from build123d import *

# Parameters (mm, degrees)
BOSS_EXTRUDE1_DEPTH = 914.4
SKETCH2_W           = 1116.884471925
SKETCH2_H           = 814.4
CUT_EXTRUDE1_DEPTH  = 19950.853735504
BOSS_EXTRUDE3_DEPTH = 850


with BuildPart() as part:
    # Sketch1 → Boss-Extrude1 (new body)
    with BuildSketch(Plane(origin=(0, 0, 0), x_dir=(1, 0, 0), z_dir=(0, 1, 0))):
        with BuildLine():
            Line((-9820.644594144, 1216.884471925), (-9871.125792152, 1216.884471925))
            ThreePointArc((-9871.125792152, 1216.884471925), (-9927.151370921, 609.588288366), (-9945.85, 0))
            Line((-9945.85, 0), (-9895.75, 0))
            ThreePointArc((-9895.75, 0), (-9876.955801384, 609.6), (-9820.644594144, 1216.884471925))
        make_face()
    extrude(amount=BOSS_EXTRUDE1_DEPTH)

    # Sketch2 → Cut-Extrude1 (cut, through all)
    with BuildSketch(Plane(origin=(9945.85, 0, 0), x_dir=(0, 0, -1), z_dir=(1, 0, 0))):
        with Locations((608.442235963, 457.2)):
            Rectangle(SKETCH2_W, SKETCH2_H)
    extrude(amount=-CUT_EXTRUDE1_DEPTH, mode=Mode.SUBTRACT)

    # Sketch5 → Boss-Extrude3 (add)
    with BuildSketch(Plane.XZ.offset(-864.4)):
        Polygon((-9925.583865068, -634.6), (-9875.381051003, -634.6), (-9878.46703201, -584.6), (-9928.654242268, -584.6), align=None)
    extrude(amount=BOSS_EXTRUDE3_DEPTH)


solid = part.part
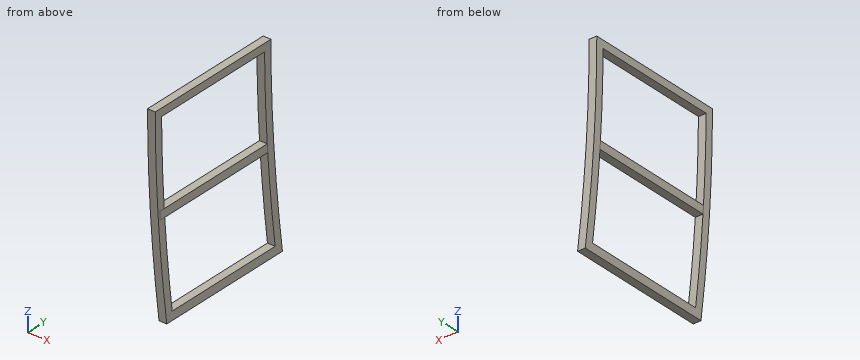
Model file for the job. Use its own axes, mm. Round coordinates to 2 decimals unless told otherwise and drop trailing zeros. Loops run counter-clockwise (first coordinate to the right, second up) from the corner with the lowest first, then second, coordinate; pieces in that order, holes last. Notation, with made-up numbers: (-26, -15) -> (-7, -15) arc R27 ccw to (-7, 5) -> close; hole circle Ø11 at (64, 74). An arc over 180 degrees is marked (long way). Answer as CSV lines item,"result". Start each with the question number.
1) Pin check, flat tips, straight feed: P1, Ø2, axis at x = -9913.5, y = 667, coming from the -Z side; P2, Ø6, axis at x = -9844, y = 622.5, coming from the +Z side. Stop position of each tip, or through.
2) Probe line 1 along Y through (x, z) = (-9888, -1005); line 2 along Z through (x, y) = (-9913, 611); line 3 along Z through (x, y) = (-9871, 562). List the from-to ranges inside material, lowest first.
3) Slice it at B-B (z = -265.5). List the corners of the cut face in (x, y).
4) Slice it at D-D (z = -77). List the corners of the cut face in (x, y), plus the area to 3 significant figures.
5) Slice it at C-C (x = -9854.5). List the corners of the cut face in (y, z), plus the area to 3 significant figures.
6) Slice it at A-A (y = 763.5). List the corners of the cut face in (x, z), plus the area to 3 significant figures.
Filled in:
1,P1,"stops at z = -634.6"
1,P2,"stops at z = -1166.88"
2,line 1,"y = 0 to 50, 864.4 to 914.4"
2,line 2,"z = -634.6 to -584.6, -50 to 0"
2,line 3,"z = -1216.88 to -1166.88"
3,outline,"(-9942.31, 0) -> (-9892.19, 0) -> (-9892.19, 50) -> (-9942.31, 50) -> close; (-9942.31, 864.4) -> (-9892.19, 864.4) -> (-9892.19, 914.4) -> (-9942.31, 914.4) -> close"
4,outline,"(-9945.55, 0) -> (-9895.45, 0) -> (-9895.45, 50) -> (-9945.55, 50) -> close; (-9945.55, 864.4) -> (-9895.45, 864.4) -> (-9895.45, 914.4) -> (-9945.55, 914.4) -> close"
4,area,"5,010 mm2"
5,outline,"(0, -1216.88) -> (914.4, -1216.88) -> (914.4, -902.61) -> (864.4, -902.61) -> (864.4, -1166.88) -> (50, -1166.88) -> (50, -902.61) -> (0, -902.61) -> close"
5,area,"72,100 mm2"
6,outline,"(-9945.85, 0) arc R9945.85 ccw to (-9945.72, -50) -> (-9895.62, -50) arc R9895.75 cw to (-9895.75, 0) -> close; (-9928.65, -584.6) -> (-9925.58, -634.6) -> (-9875.38, -634.6) -> (-9878.47, -584.6) -> close; (-9877.16, -1166.88) arc R9945.85 ccw to (-9871.13, -1216.88) -> (-9820.64, -1216.88) arc R9895.75 cw to (-9826.71, -1166.88) -> close"
6,area,"7,540 mm2"
